from build123d import *

# Parameters (mm, degrees)
F0_W     = 596.9
F0_H     = 254
F1_DEPTH = 36.576
F2_W     = 596.9
F2_H     = 290.576
F3_DEPTH = 3.175
F4_W     = 152.4
F4_H     = 25.4
F4_W_2   = 25.4
F4_H_2   = 152.4
F5_DEPTH = 6.35


with BuildPart() as f1:
    # F0 (on Right) → F1 (new body)
    with BuildSketch(Plane.YZ):
        Rectangle(F0_W, F0_H)
    extrude(amount=F1_DEPTH)

    # F2 (on face) → F3 (join)
    with BuildSketch(Plane.YZ.offset(36.576)):
        with Locations((0, -18.288)):
            Rectangle(F2_W, F2_H)
    extrude(amount=F3_DEPTH)

    # F4 (on face) → F5 (join)
    with BuildSketch(Plane.YZ.offset(39.751)):
        with Locations((152.4, 101.6)):
            Rectangle(F4_W, F4_H)
        with Locations((-260.35, 0)):
            Rectangle(F4_W_2, F4_H_2)
        with Locations((-152.4, 101.6)):
            Rectangle(F4_W, F4_H)
    extrude(amount=F5_DEPTH)


solid = f1.part
The model under review builds one solid part; all positions refer to its coordinate system, in mm. A direction names the side the tool comes from. Give positions to 0.01 mm unless a question says otherwise; leave off trailing zeros. Order: outer loops, then holes, each group sorted by start corner. A loop starts at its lowest first (then second) coordinate and runs counter-clockwise, first axis right, second up. Notation, with made-up numbers: (84, 39) -> (105, 39) arc R25 cw to (105, 69) -> close; hole circle Ø6 at (65.5, 30). An arc over 180 degrees is marked (long way). Write item = value, one per line. Start each with the question number.
(1) For pin 1 Ø5 at (x, y) = (43.5, 138) entering from +Z; pin 2 Ø5 at (x, y) = (43.5, -156) entering from -Z; pin 3 Ø4 at (x, y) = (10, 57) entering from -Z; pin 4 Ø7 at (x, y) = (43, -263.5) entering from -Z, all flat-tipped, find the tip position at first contact; note any pin that passes through.
(2) Take a section at C-C (x = 28.5). Write out the cut boundary in (y, z), plus the area to 3 significant figures.
(3) Take a section at A-A (y = -185.5). Write out the cut boundary in (x, z).
(4) Take a section at B-B (z = 67.5). Write out the cut boundary in (x, y), plus the area to 3 significant figures.
(5) Take a section at D-D (y = 253.5). Write out the cut boundary in (x, z).
(6) Tool access review of faces 1 (the flat face through (20, -298.45, -20)), 2 (the flat face through (18, -4, -127)): name each direction out of +Z, -Z, +X, -X, +Y, -Y from which nothing blocks a thin tool from reaching the whole face with its end or side.
(7) For L1, parallel to Y at x = 44.5, z = 99.5; L2, parallel to X at y = -22.5, z = 71.5; L3, parallel to Z at x = 24.5, y = 77.5, list the stretches that pass through material, from the lowest coordinate up. Write a range as from..to.
Returned:
q1.pin_1 = 114.3
q1.pin_2 = 88.9
q1.pin_3 = -127
q1.pin_4 = -163.58
q2.outline = (-298.45, -127) -> (298.45, -127) -> (298.45, 127) -> (-298.45, 127) -> close
q2.area = 152,000 mm²
q3.outline = (0, -127) -> (36.58, -127) -> (36.58, -163.58) -> (39.75, -163.58) -> (39.75, 88.9) -> (46.1, 88.9) -> (46.1, 114.3) -> (39.75, 114.3) -> (39.75, 127) -> (0, 127) -> close
q4.outline = (0, -298.45) -> (39.75, -298.45) -> (39.75, -273.05) -> (46.1, -273.05) -> (46.1, -247.65) -> (39.75, -247.65) -> (39.75, 298.45) -> (0, 298.45) -> close
q4.area = 23,900 mm²
q5.outline = (0, -127) -> (36.58, -127) -> (36.58, -163.58) -> (39.75, -163.58) -> (39.75, 127) -> (0, 127) -> close
q6.face_1 = +Z, -Z, +X, -X, -Y
q6.face_2 = -Z, -X, +Y, -Y
q7.L1 = -228.6..-76.2, 76.2..228.6
q7.L2 = 0..39.75
q7.L3 = -127..127
